Source: three-view drawing plus pictorial views. Frame: mm from the lowest corner of the part. Give positions to 0.01 mm unless a question says otherwise; leave off trailing zeros. Loops run counter-clockwise (first coordinate to the right, second up) from the corner with the lowest first, then second, coordinate; pieces in that order, holes last.
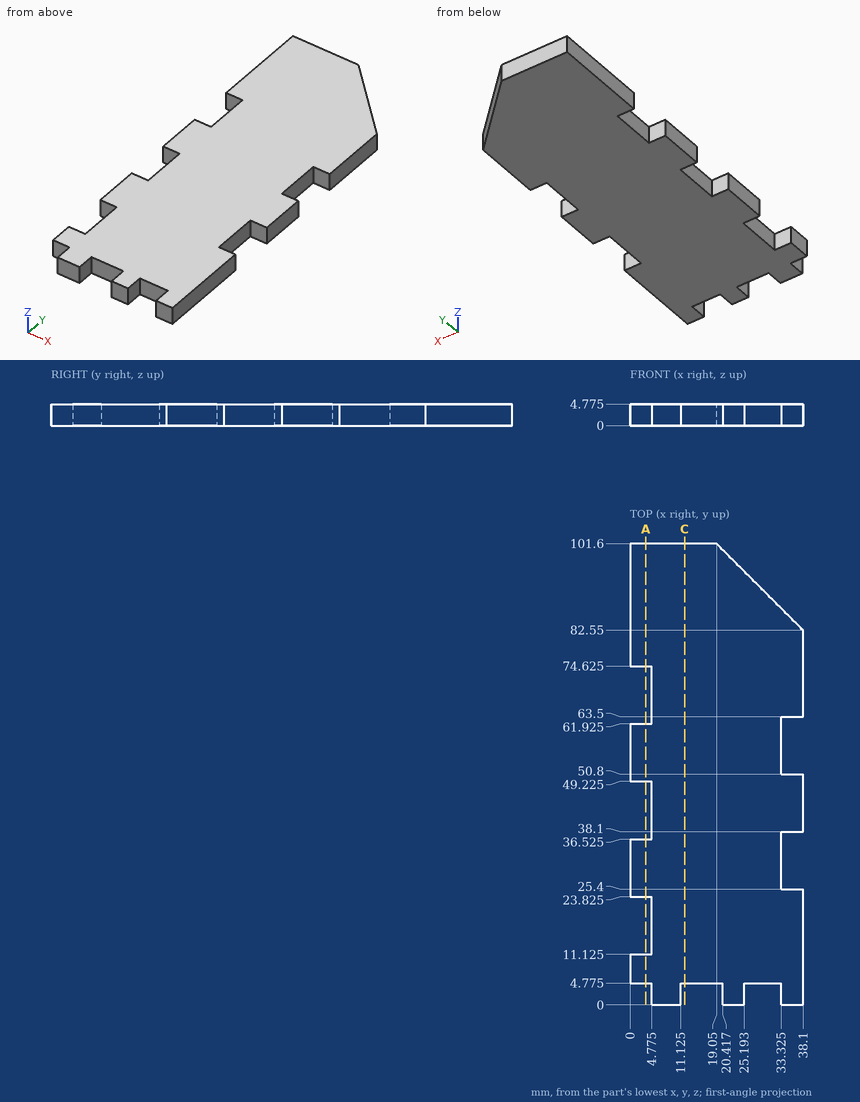
(1) Ray query, probe 1 along Y at (x, z) = (34, 4.4); probe 2 along Y at (x, z) = (12, 2.9) (1 decimal); probe 3 along X at (y, z) = (12, 3.2) (1 decimal). Return the intervals inside material, ascending.
Values follow:
probe 1: y = 0 to 25.4, 38.1 to 50.8, 63.5 to 86.65
probe 2: y = 4.8 to 101.6
probe 3: x = 4.8 to 38.1
(2) Cut plane C-C (x = 12). Return the cut outline in (y, z) (1 decimal).
Values follow:
outline: (4.8, 0) - (101.6, 0) - (101.6, 4.8) - (4.8, 4.8) - close
(3) Cut plane A-A (x = 3.5). Return the cut outline in (y, z) (1 decimal).
Values follow:
outline: (4.8, 0) - (11.1, 0) - (11.1, 4.8) - (4.8, 4.8) - close; (23.8, 0) - (36.5, 0) - (36.5, 4.8) - (23.8, 4.8) - close; (49.2, 0) - (61.9, 0) - (61.9, 4.8) - (49.2, 4.8) - close; (74.6, 0) - (101.6, 0) - (101.6, 4.8) - (74.6, 4.8) - close
(4) Pin query (flat end, axial travel): pin 1 Ø2.5 at (y, z) = (55, 1.5) entering from +X (1 decimal); pin 2 Ø2.5 at (x, z) = (3, 1.5) entering from -Y (1 decimal). Return the tip coordinate at first contact, or that it passes through.
Values follow:
pin 1: stops at x = 33.3
pin 2: stops at y = 4.8
